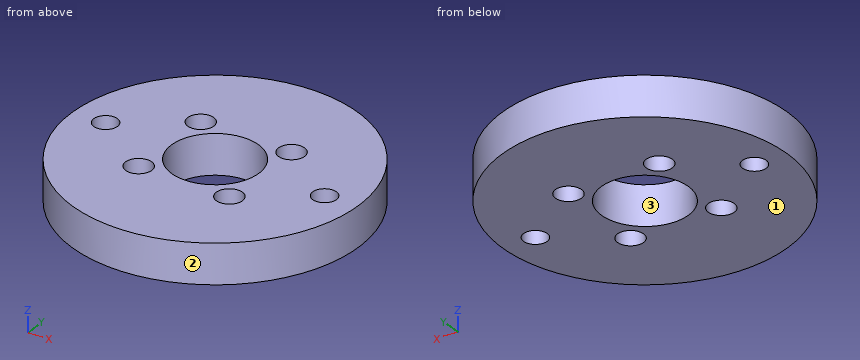
```python
from build123d import *

# Parameters (mm, degrees)
F1_DEPTH = 5
F2_D     = 3
F2_DEPTH = 6
F2_TIP   = 0.9012909285
F3_D     = 3.3
F3_DEPTH = 6
F3_TIP   = 0.9914200214
F4_D     = 11
F4_DEPTH = 11
F4_TIP   = 3.3047334047


with BuildPart() as f1:
    # F0 (on Top) → F1 (new body)
    with BuildSketch(Plane.XY):
        with BuildLine():
            Line((9.75, 0), (18, 0))
            ThreePointArc((18, 0), (0, 18), (-18, 0))
            Line((-18, 0), (-9.75, 0))
            ThreePointArc((-9.75, 0), (0, 9.75), (9.75, 0))
        make_face()
        with BuildLine():
            ThreePointArc((-18, 0), (0, -18), (18, 0))
            Line((18, 0), (9.75, 0))
            ThreePointArc((9.75, 0), (0, -9.75), (-9.75, 0))
            Line((-9.75, 0), (-18, 0))
        make_face()
        with BuildLine():
            ThreePointArc((-9.75, 0), (0, -9.75), (9.75, 0))
            ThreePointArc((9.75, 0), (0, 9.75), (-9.75, 0))
        make_face()
    extrude(amount=F1_DEPTH)

    # F2
    with Locations(Plane(origin=(0, 0, 0), x_dir=(1, 0, 0), z_dir=(0, 0, -1))):
        with Locations((13.875, 0), (-13.875, 0)):
            Hole(F2_D / 2, depth=F2_DEPTH)
            with Locations((0, 0, -(F2_DEPTH + F2_TIP / 2))):  # 118° drill point
                Cone(0, F2_D / 2, F2_TIP, mode=Mode.SUBTRACT)

    # F3
    with Locations(Plane(origin=(0, 0, 0), x_dir=(1, 0, 0), z_dir=(0, 0, -1))):
        with Locations((5.75, -5.75), (5.75, 5.75), (-5.75, 5.75), (-5.75, -5.75)):
            Hole(F3_D / 2, depth=F3_DEPTH)
            with Locations((0, 0, -(F3_DEPTH + F3_TIP / 2))):  # 118° drill point
                Cone(0, F3_D / 2, F3_TIP, mode=Mode.SUBTRACT)

    # F4
    with Locations(Plane(origin=(0, 0, 0), x_dir=(1, 0, 0), z_dir=(0, 0, -1))):
        with Locations((0, 0)):
            Hole(F4_D / 2, depth=F4_DEPTH)
            with Locations((0, 0, -(F4_DEPTH + F4_TIP / 2))):  # 118° drill point
                Cone(0, F4_D / 2, F4_TIP, mode=Mode.SUBTRACT)


solid = f1.part
```
CAD build for the part. Positions are in the model's coordinates, mm. Face numbers are marked on the shaded views. Round coordinates to 2 decimals unless told otherwise and drop trailing zeros. Write each loop counter-clockwise with the first axis right and the second up, starting at its lowest first coordinate (ties: lowest second). Pieces come first, ordered by that corner, then holes.
Item 1: Band-saw the part on D-D on y = -11. Write the cut outline in (x, z), then the cut area to 3 significant figures.
Filled in:
outline: (-14.25, 0) - (14.25, 0) - (14.25, 5) - (-14.25, 5) - close
area: 142 mm2
Item 2: Band-saw the part on A-A on z = 3.05. Write the cut outline in (x, y) (3 decimals).
Filled in:
outline: circle Ø36 at (0, 0); hole circle Ø3 at (-13.875, 0); hole circle Ø3.3 at (-5.75, -5.75); hole circle Ø3.3 at (-5.75, 5.75); hole circle Ø11 at (0, 0); hole circle Ø3.3 at (5.75, -5.75); hole circle Ø3.3 at (5.75, 5.75); hole circle Ø3 at (13.875, 0)
Item 3: Band-saw the part on C-C on x = 0. Write the cut outline in (y, z).
Filled in:
outline: (-18, 0) - (-5.5, 0) - (-5.5, 5) - (-18, 5) - close; (5.5, 0) - (18, 0) - (18, 5) - (5.5, 5) - close
Item 4: Band-saw the part on B-B on y = 0. Write the cut outline in (x, z) (3 decimals).
Filled in:
outline: (-18, 0) - (-15.375, 0) - (-15.375, 5) - (-18, 5) - close; (-12.375, 0) - (-5.5, 0) - (-5.5, 5) - (-12.375, 5) - close; (5.5, 0) - (12.375, 0) - (12.375, 5) - (5.5, 5) - close; (15.375, 0) - (18, 0) - (18, 5) - (15.375, 5) - close
Item 5: Drop flat-ended pins along their axis: pin 1 Ø1 at (x, z) = (-9, 1.5) entering from +Y; pin 2 Ø5.5 at (x, y) = (5.75, 5.75) entering from +Z; pin 3 Ø2 at (x, z) = (-7.5, 4.5) entering from -Y; pin 4 Ø2 at (x, y) = (-5.75, -5.75) entering from -Z. Give the stop position or say it passes through.
Filled in:
pin 1: stops at y = 15.87
pin 2: stops at z = 5
pin 3: stops at y = -16.79
pin 4: passes through
Item 6: Drill centre lines: L1, parallel to X at y = 4.5, z = 4.4; L2, parallel to X at y = -6.5, z = 3.8; L3, parallel to Y at x = -5.75, z = 3.75. Where is each one in solid material? Low to high.
Filled in:
L1: x = -17.43 to -6.83, -4.67 to -3.16, 3.16 to 4.67, 6.83 to 17.43
L2: x = -16.79 to -7.22, -4.28 to 4.28, 7.22 to 16.79
L3: y = -17.06 to -7.4, -4.1 to 4.1, 7.4 to 17.06
Item 7: Mould opens along Y. For the marked faces 1, 2 and 3 say: released by +Y, released by -Y, zero draft, split by the parting line, or undercut.
Filled in:
face 1: zero draft
face 2: split by the parting line
face 3: undercut
